Solid Edge part; units mm, degrees
sketch "Sketch1" plane through (0, 0, 0) normal (0, 0, 1) x (1, 0, 0)
  line L0 (0, -70.7107) -> (70.7107, 0)
  line L1 (70.7107, 0) -> (0, 70.7107)
  line L2 (0, 70.7107) -> (-70.7107, 0)
  line L3 (-70.7107, 0) -> (0, -70.7107)
extrude "Protrusion1" add sketch "Sketch1" along normal up to vertex (70.7107 mm away)
sketch "Sketch2" plane through (-35.3553, -35.3553, 35.3553) normal (-0.7071, -0.7071, 0) x (0.7071, -0.7071, 0)
  line L0 (0, 35.3553) -> (50, -35.3553)
extrude "Cutout1" cut sketch "Sketch2" against normal up to next material side at (-17.6488, -53.0618, 35.3842)
pattern_circular "Pattern1" count 4 over 360 about axis through (0, 0, 70.7107) along (0, 0, -1) of "Cutout1"
Geometry: final body of the model. Coordinates: model frame, mm. Give positions to 0.01 mm unless a question says otherwise; leave off trailing zeros. Loops run counter-clockwise (first coordinate to the right, second up) from the corner with the lowest first, then second, coordinate; pieces in that order, holes last. Notation, with made-up numbers: (7, 33.5) - (58, 33.5) arc R9 ccw to (58, 45.5) - close; hole circle Ø7 at (14, -29.5). An arc over 180 degrees is marked (long way). One line per question, with ' | ' between items. Start each with the question number.
(1) Section query A-A on x = -11.5. Return loops of the section in (y, z).
(2) Section query B-B on z = 16. Return loops of the section in (x, y), then the cut area to 3 significant figures.
(3) Ray query, line 1 (Y direction, x = -14, z = 46); line 2 (Z direction, x = 41.5, y = 7); line 3 (Y direction, x = 3.5, z = 27.5). Return the intervals inside material, ascending. Write a range as from..to.
(4) Contact query for flat-ended pins moving along their axis: pin 1 (6 mm diameter, centred on x = -18.5, z = 54, fed in from -Y); pin 2 (10 mm diameter, centred on x = 42, y = 5.5, fed in from +Z); pin 3 (10 mm diameter, centred on x = -45.5, z = 21, fed in from -Y). Output: stop coordinate, or through.
(5) Section query C-C on y = -41. Return loops of the section in (x, z), then the cut area to 3 significant figures.
(6) Section query D-D on z = 52. Return loops of the section in (x, y).
The answers:
1) outline: (-59.21, 0) - (59.21, 0) - (0, 59.21) - close
2) outline: (-54.71, 0) - (0, -54.71) - (54.71, 0) - (0, 54.71) - close | area: 5,990 mm2
3) line 1: -10.71..10.71 | line 2: 0..22.21 | line 3: -39.71..39.71
4) pin 1: y = -2.45 | pin 2: z = 30.28 | pin 3: y = -11.28
5) outline: (-29.71, 0) - (29.71, 0) - (0, 29.71) - close | area: 883 mm2
6) outline: (-18.71, 0) - (0, -18.71) - (18.71, 0) - (0, 18.71) - close
